Verification items for the finished model (mm, model axes). Give positions to 0.01 mm unless a question says otherwise; leave off trailing zeros. Write each loop counter-clockwise with the first axis right and the second up, starting at its lowest first coordinate (ties: lowest second). Pieces come first, ordered by that corner, then holes. Notation, with made-up numbers: (36.25, -29.75) - (64.25, -29.75) arc R19 ccw to (64.25, -22.75) - close; hole circle Ø4 at (76, -31). An arc over 180 degrees is marked (long way). Answer as a JSON object with one key per item and string values. Group by question number.
Item 1: Go/stop test with flat-tipped pins: pin 1 (1.5 mm diameter, centred on y = 9, z = -3, fed in from +X); pin 2 (6 mm diameter, centred on y = 14, z = 4, fed in from +X). Record where each tip stops, or that it passes through.
Item 2: Draft check along X on faces 1 (the face through (-5.994, -7.582, 0.264)), 2 (the face through (-3, 17.875, 3)), 3 (the face through (1.03, -0.25, 3.27)). Enter one of: +X half, -X half, draft (parallel to the pull), parting line (faces both ways), or undercut.
Item 3: Sectioned sample at B-B, the plane x = 0. Record the boundary of the cut face in (y, z) (3 decimals), and give its area (3 significant figures).
Item 4: Scan lines: line 1 along X through (y, z) = (-2.5, 0) (3 decimals); line 2 along Y through (x, z) = (-5.5, -2.5) (3 decimals); line 3 along X through (y, z) = (-13, 1.25). Record each from-to range of solid material in increasing order. Write a range as [from, to].
Item 5: Sectioned sample at D-D, the plane z = -4.5. Record the boundary of the cut face in (x, y) (3 decimals).
Item 6: Sectioned sample at C-C, the plane y = -2.5. Record the boundary of the cut face in (x, z) (3 decimals), and give its area (3 significant figures).
Item 7: Sectioned sample at A-A, the plane z = 2.25. Record the boundary of the cut face in (x, y) (3 decimals), and give its area (3 significant figures).
```python
from build123d import *

# Parameters (mm, degrees)
SKETCH1_R               = 6.125
SKETCH1_R_2             = 3.43
BOSS_EXTRUDE1_DEPTH     = 17.875
CUT_EXTRUDE_THIN1_START = -9.8
SKETCH2_R               = 6.5
SKETCH2_R_2             = 6
CUT_EXTRUDE_THIN1_DEPTH = 1


with BuildPart() as part:
    # Sketch1 → Boss-Extrude1 (new, symmetric)
    with BuildSketch(Plane(origin=(0, 0, 0), x_dir=(1, 0, 0), z_dir=(0, 1, 0))):
        with Locations(Location((0, 0, 0), (0, 0, 270))):
            Circle(SKETCH1_R)
        with Locations(Location((0, 0, 0), (0, 0, 270))):
            Circle(SKETCH1_R_2, mode=Mode.SUBTRACT)
    extrude(amount=BOSS_EXTRUDE1_DEPTH, both=True)

    # Sketch2 → Cut-Extrude-Thin1 (cut)
    with BuildSketch(Plane.XZ.offset(17.875).offset(CUT_EXTRUDE_THIN1_START)):
        Circle(SKETCH2_R)
        Circle(SKETCH2_R_2, mode=Mode.SUBTRACT)
    extrude(amount=-CUT_EXTRUDE_THIN1_DEPTH, mode=Mode.SUBTRACT)


solid = part.part
```
Geometry check:
{
 "1": {"pin 1": "x = 5.7", "pin 2": "x = 6.04"},
 "2": {"face 1": "parting line", "face 2": "draft", "face 3": "undercut"},
 "3": {"outline": "(-17.875, -6.125) - (-8.075, -6.125) - (-8.075, -6) - (-7.075, -6) - (-7.075, -6.125) - (17.875, -6.125) - (17.875, -3.43) - (-17.875, -3.43) - close; (-17.875, 3.43) - (17.875, 3.43) - (17.875, 6.125) - (-7.075, 6.125) - (-7.075, 6) - (-8.075, 6) - (-8.075, 6.125) - (-17.875, 6.125) - close", "area": "192 mm^2"},
 "4": {"line 1": "[-6.125, -3.43], [3.43, 6.125]", "line 2": "[-17.875, -8.075], [-7.075, 17.875]", "line 3": "[-6, -3.19], [3.19, 6]"},
 "5": {"outline": "(-4.155, -17.875) - (4.155, -17.875) - (4.155, -8.075) - (3.969, -8.075) - (3.969, -7.075) - (4.155, -7.075) - (4.155, 17.875) - (-4.155, 17.875) - (-4.155, -7.075) - (-3.969, -7.075) - (-3.969, -8.075) - (-4.155, -8.075) - close"},
 "6": {"outline": "circle Ø12.25 at (0, 0); hole circle Ø6.86 at (0, 0)", "area": "80.9 mm^2"},
 "7": {"outline": "(-5.697, -17.875) - (-2.589, -17.875) - (-2.589, 17.875) - (-5.697, 17.875) - (-5.697, -7.075) - (-5.562, -7.075) - (-5.562, -8.075) - (-5.697, -8.075) - close; (2.589, -17.875) - (5.697, -17.875) - (5.697, -8.075) - (5.562, -8.075) - (5.562, -7.075) - (5.697, -7.075) - (5.697, 17.875) - (2.589, 17.875) - close", "area": "222 mm^2"}
}
